Geometry: final body of the model. Coordinates: model frame, mm. Face numbers are marked on the shaded views. Round coordinates to 2 decimals unless told otherwise and drop trailing zeros. Loops run counter-clockwise (first coordinate to the right, second up) from the corner with the lowest first, then second, coordinate; pieces in that order, holes last. Notation, with made-up numbers: M -12,9 L 15,9 A17 ccw 15,21 Z; hole C -6.5,68 d2. An arc over 180 degrees is marked long. Return JSON: item names as keys, results as strings.
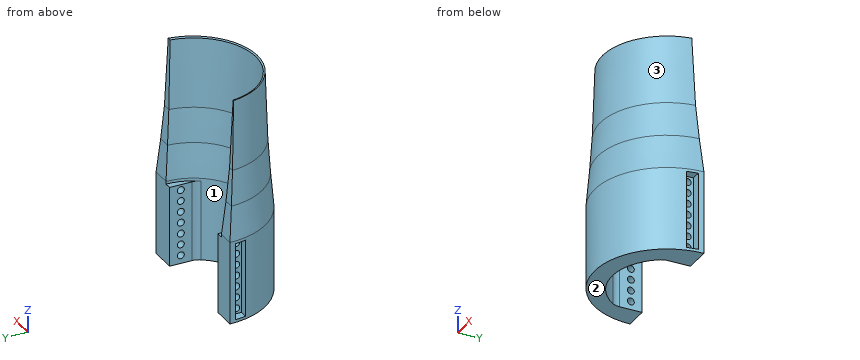
from build123d import *

# Parameters (mm, degrees)
BOSS_EXTRUDE1_DEPTH     = 60
BOSS_EXTRUDE2_DEPTH     = 25
BOSS_EXTRUDE2_TAPER     = 5
BOSS_EXTRUDE3_DEPTH     = 25
BOSS_EXTRUDE3_TAPER     = 4
BOSS_EXTRUDE4_DEPTH     = 50
BOSS_EXTRUDE4_TAPER     = 2
SKETCH5_W               = 5
SKETCH5_H               = 30
BOSS_EXTRUDE5_DEPTH     = 58
FILLET1_R               = 10
CUT_EXTRUDE1_DEPTH      = 189.491379271
CUT_EXTRUDE1_DEPTH_BACK = 189.491379271
SKETCH6_R               = 2.5
CUT_EXTRUDE2_START      = -10
SKETCH7_W               = 56
SKETCH7_H               = 8
CUT_EXTRUDE2_DEPTH      = 58


with BuildPart() as part:
    # Sketch1 → Boss-Extrude1 (new body)
    with BuildSketch(Plane.XY):
        with BuildLine():
            ThreePointArc((38, 0), (-1, -39), (-40, 0))
            Line((-40, 0), (-52, 0))
            ThreePointArc((-52, 0), (0, -52), (52, 0))
            Line((52, 0), (38, 0))
        make_face()
    extrude(amount=BOSS_EXTRUDE1_DEPTH)

    # Sketch2 → Boss-Extrude2 (add)
    with BuildSketch(Plane.XY.offset(60)):
        with BuildLine():
            Line((-40, 0), (-52, 0))
            ThreePointArc((-52, 0), (0, -52), (52, 0))
            Line((52, 0), (38, 0))
            ThreePointArc((38, 0), (-1, -39), (-40, 0))
        make_face()
    extrude(amount=BOSS_EXTRUDE2_DEPTH, taper=BOSS_EXTRUDE2_TAPER)

    # Sketch3 → Boss-Extrude3 (add)
    with BuildSketch(Plane.XY.offset(85)):
        with BuildLine():
            Line((-42.129100329, -2.187216588), (-49.764741282, -2.187216588))
            ThreePointArc((-49.764741282, -2.187216588), (0, -49.812783412), (49.764741282, -2.187216588))
            Line((49.764741282, -2.187216588), (40.129100329, -2.187216588))
            ThreePointArc((40.129100329, -2.187216588), (-1, -41.187216588), (-42.129100329, -2.187216588))
        make_face()
    extrude(amount=BOSS_EXTRUDE3_DEPTH, taper=BOSS_EXTRUDE3_TAPER)

    # Sketch4 → Boss-Extrude4 (add)
    with BuildSketch(Plane.XY.offset(110)):
        with BuildLine():
            Line((-43.754650942, -3.935386887), (-47.903233333, -3.935386887))
            ThreePointArc((-47.903233333, -3.935386887), (0, -48.064613113), (47.903233333, -3.935386887))
            Line((47.903233333, -3.935386887), (41.754650942, -3.935386887))
            ThreePointArc((41.754650942, -3.935386887), (-1, -42.935386887), (-43.754650942, -3.935386887))
        make_face()
    extrude(amount=BOSS_EXTRUDE4_DEPTH, taper=BOSS_EXTRUDE4_TAPER)

    # Sketch5 → Boss-Extrude5 (add)
    with BuildSketch(Plane(origin=(0, 0, 0), x_dir=(-1, 0, 0), z_dir=(0, 0, -1))):
        with Locations((-35.5, -15)):
            Rectangle(SKETCH5_W, SKETCH5_H)
        with Locations((37.5, -15)):
            Rectangle(SKETCH5_W, SKETCH5_H)
    extrude(amount=-BOSS_EXTRUDE5_DEPTH)

    # Fillet1
    fillet1_edges = [part.edges().sort_by_distance(p)[0] for p in [
        (33, -19.104973175, 29),
        (-35, -19.104973175, 29),
    ]]
    fillet(fillet1_edges, radius=FILLET1_R)

    # Sketch6 → Cut-Extrude1 (cut, two sides: drawn at the far end of the back side and taken through both)
    with BuildSketch(Plane.ZY.offset(-33).offset(-CUT_EXTRUDE1_DEPTH_BACK)):
        with Locations(Location((6, -8.14, 0), (0, 0, 270))):
            Circle(SKETCH6_R)
        with Locations(Location((14, -8.14, 0), (0, 0, 270))):
            Circle(SKETCH6_R)
        with Locations(Location((22, -8.14, 0), (0, 0, 270))):
            Circle(SKETCH6_R)
        with Locations(Location((30, -8.14, 0), (0, 0, 270))):
            Circle(SKETCH6_R)
        with Locations(Location((38, -8.14, 0), (0, 0, 270))):
            Circle(SKETCH6_R)
        with Locations(Location((46, -8.14, 0), (0, 0, 270))):
            Circle(SKETCH6_R)
        with Locations(Location((54, -8.14, 0), (0, 0, 270))):
            Circle(SKETCH6_R)
    extrude(amount=CUT_EXTRUDE1_DEPTH + CUT_EXTRUDE1_DEPTH_BACK, mode=Mode.SUBTRACT)

    # Sketch7 → Cut-Extrude2 (cut)
    with BuildSketch(Plane(origin=(-35, 0, 0), x_dir=(0, 0, -1), z_dir=(1, 0, 0)).offset(CUT_EXTRUDE2_START)):
        with Locations((-30, -8)):
            Rectangle(SKETCH7_W, SKETCH7_H)
    cut_extrude2 = extrude(amount=-CUT_EXTRUDE2_DEPTH, mode=Mode.SUBTRACT)

    # Mirror1: Cut-Extrude2 across plane
    add(cut_extrude2.mirror(Plane(origin=(0, 0, 0), x_dir=(0, 0, 1), z_dir=(1, 0, 0))), mode=Mode.SUBTRACT)


solid = part.part
Q1. Pull-direction query (X, two-part tool) for the marked faces 1, 2 and 3; classes: pulls with the +X half, pulls with the -X half, needs draft (parallel to the pull), parting line crosses it, or undercut.
Determined:
{"face 1": "undercut", "face 2": "needs draft", "face 3": "parting line crosses it"}
Q2. Section query D-D (z = 106.5). Output: boundary loops of the cut face in (x, y).
Determined:
{"outline": "M -48.17,-3.69 A48.31 ccw 48.17,-3.69 L 41.53,-3.69 A42.69 cw -43.53,-3.69 Z"}
Q3. Material intervals for L1, parallel to X at y = -6.5, z = 24; L2, parallel to X at y = -21, z = 71; L3, parallel to Y at x = -37.25, z = 14, sorted ascending.
Determined:
{"L1": "x = -45 to -35, 33 to 45", "L2": "x = -46.52 to -35, 33 to 46.52", "L3": "y = -36.28 to -10.64, -5.64 to 0"}
Q4. Section query B-B (y = -8.14). State how many separate pieces and enclosed holes the cut face has, plus the area to 3 significant figures.
Determined:
{"separate pieces": "16", "enclosed holes": "0", "area": "1,830 mm^2"}
Q5. Section query A-A (z = 54). Output: boundary loops of the cut face in (x, y), plus the area to 3 significant figures.
Determined:
{"outline": "M -52,0 A52 ccw -51.85,-4 L -45,-4 L -45,-5.64 L -35,-5.64 L -35,0 Z; M -50.6,-12 A52 ccw 50.6,-12 L 45,-12 L 45,-10.64 L 33,-10.64 L 33,-16.28 A10 cw 31.28,-21.89 A39 cw -33.28,-21.89 A10 cw -35,-16.28 L -35,-10.64 L -45,-10.64 L -45,-12 Z; M 33,-5.64 L 45,-5.64 L 45,-4 L 51.85,-4 A52 ccw 52,0 L 33,0 Z", "area": "1,780 mm^2"}
Q6. Pin query (flat end, axial travel): pin 1 (2 mm diameter, centred on x = -48, z = 16.5, fed in from -Y); pin 2 (1.5 mm diameter, centred on x = 33.5, z = 17, fed in from -Y); pin 3 (6.5 mm diameter, centred on y = -8.14, z = 54, fed in from -X). Return the tip coordinate at first contact, or that it passes through.
Determined:
{"pin 1": "stops at y = -22.25", "pin 2": "stops at y = -40.39", "pin 3": "stops at x = -45"}
